Check sheet for the modelled part. Datum: model origin and axes. Units: mm. A direction names the side the tool comes from. Round coordinates to 2 decimals unless told otherwise and drop trailing zeros. Write each loop counter-clockwise with the first axis right and the second up, starting at its lowest first coordinate (ties: lowest second). Pieces come first, ordered by that corner, then holes.
Item 1: Material ranges on line 1 (Z direction, x = -63, y = 6.25); line 2 (X direction, y = 7, z = -33); line 3 (X direction, y = 8.25, z = -10.5), recorded low to high.
Item 2: Cross-section at A-A on x = 63. Enter the section's corners in (y, z).
Item 3: Tool access check on faces 4 (the flat face through (59, 6, -20)), 5 (the flat face through (-19, 6, 40)), 6 (the flat face through (-59, 6, -20)). Record the directions out of +Z, -Z, +X, -X, +Y, -Y that give a thin tool (end or side, any length) a straight path to the whole face; none if there is none.
Item 4: Cross-section at B-B on z = 0. Enter the section's corners in (x, y), plus the area to 3 significant figures.
Item 5: Cross-section at D-D on z = -26. Enter the section's corners in (x, y), plus the area to 3 significant figures.
Item 6: Go/stop test with flat-tipped pins: pin 1 Ø2 at (x, y) = (49, 2) entering from +Z; pin 2 Ø3.5 at (y, z) = (5, 37.5) entering from -X; pin 3 Ø3.5 at (x, y) = (-55, 5.5) entering from -Z. Record where each tip stops, or that it passes through.
Item 7: Release check for a two-part mould opening along Z. For faces 1 (the flat face through (10, 11.3, -36)), 2 (the cylindrical face through (-36.877, 5.729, 38.067)), 3 (the cylindrical face through (-29.64, 5.73, 31.53)) record: +Z half, -Z half, draft (parallel to the pull), parting line (faces both ways), or undercut.
Item 8: Cross-section at C-C on y = 2. Count the separate pieces of the cut face and the enclosed holes in it, plus the area to 3 significant figures.
from build123d import *

# Parameters (mm, degrees)
SKETCH1_W                                  = 53
SKETCH1_H                                  = 11.3
SKETCH2_R                                  = 36
CUT_EXTRUDE1_DEPTH                         = 11.3
SKETCH3_W                                  = 38
SKETCH3_H                                  = 11.3
CUT_EXTRUDE2_DEPTH                         = 41.3
SKETCH5_R                                  = 2.2
CUT_EXTRUDE3_DEPTH                         = 76.800329815
CIRPATTERN1_COUNT                          = 3
BOSS_EXTRUDE1_START                        = -5
SKETCH6_W                                  = 40
SKETCH6_H                                  = 11.3
BOSS_EXTRUDE1_DEPTH                        = 22
SKETCH7_R                                  = 3.2
CUT_EXTRUDE4_DEPTH                         = 89.525081192
MIRROR2_AT_THE_SECOND_PLANE_COPY_1_SKETC_R = 3.2
MIRROR2_AT_THE_SECOND_PLANE_COPY_1_DEPTH   = 89.525081192


with BuildPart() as part:
    # Sketch1 → Revolve1 (revolve)
    with BuildSketch(Plane(origin=(0, 0, 0), x_dir=(0, 0, -1), z_dir=(1, 0, 0)), mode=Mode.PRIVATE) as revolve1_sk:
        with Locations((26.5, 5.65)):
            Rectangle(SKETCH1_W, SKETCH1_H)
    revolve(revolve1_sk.sketch.rotate(Axis((0, 28.592836715, 0), (0, -1, 0)), 180), axis=Axis((0, 28.592836715, 0), (0, -1, 0)))

    # Sketch2 → Cut-Extrude1 (cut)
    with BuildSketch(Plane(origin=(0, 11.3, 0), x_dir=(1, 0, 0), z_dir=(0, 1, 0))):
        with Locations(Location((0, 0, 0), (0, 0, 270))):
            Circle(SKETCH2_R)
    extrude(amount=-CUT_EXTRUDE1_DEPTH, mode=Mode.SUBTRACT)

    # Sketch3 → Cut-Extrude2 (cut)
    with BuildSketch(Plane.XY.offset(53)):
        with Locations((0, 5.65)):
            Rectangle(SKETCH3_W, SKETCH3_H)
    extrude(amount=-CUT_EXTRUDE2_DEPTH, mode=Mode.SUBTRACT)

    # Sketch5 → Cut-Extrude3 (cut, through all)
    with BuildSketch(Plane(origin=(0, 11.3, 0), x_dir=(1, 0, 0), z_dir=(0, 1, 0))):
        with Locations((11.64685703, -43.466662183)):
            Circle(SKETCH5_R)
        with Locations(Location((-11.64685703, 43.466662183, 0), (0, 0, 270))):
            Circle(SKETCH5_R)
    cut_extrude3 = extrude(amount=-CUT_EXTRUDE3_DEPTH, mode=Mode.SUBTRACT)

    # CirPattern1: Cut-Extrude3 ×3 about axis
    cirpattern1_axis = Axis((0, 0, 0), (0, 1, 0))
    for i in range(1, CIRPATTERN1_COUNT):
        add(cut_extrude3.rotate(cirpattern1_axis, i * 360 / CIRPATTERN1_COUNT), mode=Mode.SUBTRACT)

    # Sketch6 → Boss-Extrude1 (add)
    with BuildSketch(Plane(origin=(53, 0, 0), x_dir=(0, 0, -1), z_dir=(1, 0, 0)).offset(BOSS_EXTRUDE1_START)):
        with Locations((0, 5.65)):
            Rectangle(SKETCH6_W, SKETCH6_H)
    boss_extrude1 = extrude(amount=BOSS_EXTRUDE1_DEPTH)

    # Mirror1: Boss-Extrude1 across plane
    add(boss_extrude1.mirror(Plane(origin=(0, 0, 0), x_dir=(0, 0, 1), z_dir=(1, 0, 0))))

    # Sketch7 → Cut-Extrude4 (cut, through all)
    with BuildSketch(Plane(origin=(0, 11.3, 0), x_dir=(1, 0, 0), z_dir=(0, 1, 0))):
        with Locations(Location((63, 10.5, 0), (0, 0, 270))):
            Circle(SKETCH7_R)
    cut_extrude4 = extrude(amount=-CUT_EXTRUDE4_DEPTH, mode=Mode.SUBTRACT)

    # Mirror2: Cut-Extrude4 across plane
    add(cut_extrude4.mirror(Plane(origin=(0, 0, 0), x_dir=(0, 0, 1), z_dir=(1, 0, 0))), mode=Mode.SUBTRACT)

    # Mirror2 at the second plane: Cut-Extrude4 across plane
    add(cut_extrude4.mirror(Plane.XY), mode=Mode.SUBTRACT)

    # Mirror2 at the second plane copy 1 sketc → Mirror2 at the second plane copy 1 (cut, through all)
    with BuildSketch(Plane(origin=(0, 11.3, 0), x_dir=(-1, 0, 0), z_dir=(0, 1, 0))):
        with Locations(Location((63, 10.5, 0), (0, 0, 270))):
            Circle(MIRROR2_AT_THE_SECOND_PLANE_COPY_1_SKETC_R)
    extrude(amount=-MIRROR2_AT_THE_SECOND_PLANE_COPY_1_DEPTH, mode=Mode.SUBTRACT)


solid = part.part
Response values:
1. line 1: z = -20 to -13.7, -7.3 to 7.3, 13.7 to 20
1. line 2: x = -41.47 to -14.39, 14.39 to 29.96, 33.68 to 41.47
1. line 3: x = -70 to -66.2, -59.8 to -45.34, -41.59 to -34.43, 34.43 to 59.8, 66.2 to 70
2. outline: (0, -20) - (11.3, -20) - (11.3, -13.7) - (0, -13.7) - close; (0, -7.3) - (11.3, -7.3) - (11.3, 7.3) - (0, 7.3) - close; (0, 13.7) - (11.3, 13.7) - (11.3, 20) - (0, 20) - close
3. face 4: -Z, +X, +Y, -Y
3. face 5: +Z, +Y, -Y
3. face 6: -Z, -X, +Y, -Y
4. outline: (-70, 0) - (-36, 0) - (-36, 11.3) - (-70, 11.3) - close; (36, 0) - (70, 0) - (70, 11.3) - (36, 11.3) - close
4. area: 768 mm2
5. outline: (-46.18, 0) - (-24.9, 0) - (-24.9, 11.3) - (-46.18, 11.3) - close; (24.9, 0) - (46.18, 0) - (46.18, 11.3) - (24.9, 11.3) - close
5. area: 481 mm2
6. pin 1: stops at z = 22.47
6. pin 2: stops at x = -39.13
6. pin 3: stops at z = -20
7. face 1: draft
7. face 2: +Z half
7. face 3: undercut
8. separate pieces: 1
8. enclosed holes: 9
8. area: 5,340 mm2
